Input: part model. Units: mm. Frame: model coordinates. A direction names the side the tool comes from. Coordinates: 2 decimals unless noted, no trailing zeros. Write each loop counter-clockwise with the first axis right and the second up, starting at its lowest first coordinate (ties: lowest second). Pieces come first, ordered by that corner, then holes. Notation, with made-up numbers: M -32.75,38.5 L 2.25,38.5 A5 cw 2.25,44.5 Z; hole C 7.5,-31.5 d3. An arc over 180 degrees is marked long. Use one line per item in the form item = value.
from build123d import *

# Parameters (mm, degrees)
SKETCH1_R           = 5.05
BOSS_EXTRUDE1_DEPTH = 87
BOSS_EXTRUDE1_TAPER = 1
SKETCH2_R           = 0.5
BOSS_EXTRUDE2_DEPTH = 0.5


with BuildPart() as part:
    # Sketch1 → Boss-Extrude1 (new body)
    with BuildSketch(Plane(origin=(0, 0, 0), x_dir=(0, 0, -1), z_dir=(1, 0, 0))):
        Circle(SKETCH1_R)
    extrude(amount=BOSS_EXTRUDE1_DEPTH, taper=BOSS_EXTRUDE1_TAPER)

    # Sketch2 → Boss-Extrude2 (add, symmetric)
    with BuildSketch(Plane(origin=(0, 0, 0), x_dir=(1, 0, 0), z_dir=(0, 1, 0))):
        with BuildLine():
            Line((0, 1), (-1, 1))
            ThreePointArc((-1, 1), (-2, 0), (-1, -1))
            Line((-1, -1), (0, -1))
            Line((0, -1), (0, 1))
        make_face()
        with Locations((-1, 0)):
            Circle(SKETCH2_R, mode=Mode.SUBTRACT)
    extrude(amount=BOSS_EXTRUDE2_DEPTH, both=True)


solid = part.part
(1) Section query B-B on x = 38.5. Return the cut outline in (y, z).
Computed:
outline = C 0,0 d8.76
(2) Section query A-A on x = 51. Return the cut outline in (y, z).
Computed:
outline = C 0,0 d8.32
(3) Set-up query: faces 1 (the conical face through (44.109, 4.244, 0.557)), 2 (the flat face through (87, 0, 0)), 3 (the flat face through (-0.3, -0.5, 0)), 4 (the flat face through (-0.3, 0.5, 0)). Return all of +Z, -Z, +X, -X, +Y, -Y with unobstructed straight access to the full face (end or side cutting, diameter ignored); none if empty.
Computed:
face_1 = +X
face_2 = +Z, -Z, +X, +Y, -Y
face_3 = +Z, -Z, -X, -Y
face_4 = +Z, -Z, -X, +Y
(4) First-contact query: pin 1 Ø6 at (x, y) = (12, 0.5) entering from -Z; pin 2 Ø3 at (x, y) = (7, 0) entering from -Z; pin 3 Ø1 at (x, y) = (64.5, -2.5) entering from +Z; pin 4 Ø0.6 at (x, z) = (-1, 0) entering from -Y. Flat tips, straight axial feed; report the tip coordinate or a pass-through.
Computed:
pin_1 = -4.89
pin_2 = -4.95
pin_3 = 3.38
pin_4 = through
(5) Line query: probe 1 along Z at (x, y) = (-1, -0.2); probe 2 along X at (y, z) = (0.1, 0); probe 3 along X at (y, z) = (0.5, 1.5). Output: solid intervals per line, ascending.
Computed:
probe_1 = -1 to -0.5, 0.5 to 1
probe_2 = -2 to -1.5, -0.5 to 87
probe_3 = 0 to 87
